Build history of the part. All positions in model axes, mm. Face numbers are marked on the shaded views. A direction names the side the tool comes from. Give positions to 0.01 mm unless a question says otherwise; leave off trailing zeros. Order: outer loops, then holes, each group sorted by start corner. A loop starts at its lowest first (then second) coordinate and runs counter-clockwise, first axis right, second up. Notation, with made-up numbers: (82.5, 29) - (121.5, 29) arc R25 ccw to (121.5, 68) - close; hole circle Ø8 at (-31, 84.25). An arc over 180 degrees is marked (long way). Write each question's results on one line, items separated by ' | '. Start each with the question number.
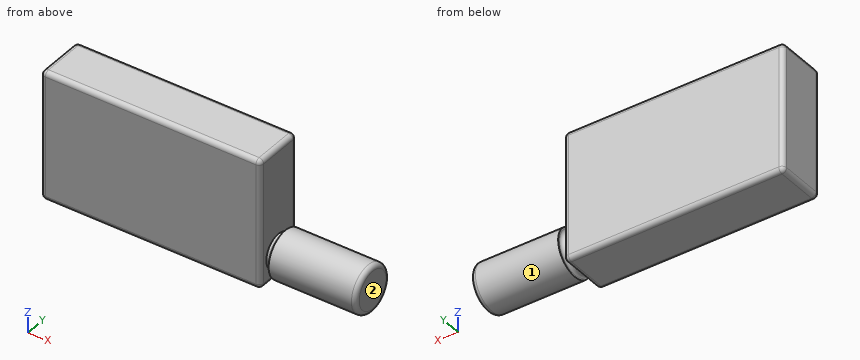
from build123d import *

# Parameters (mm, degrees)
SKETCH1_W           = 48
SKETCH1_H           = 28.2
BOSS_EXTRUDE1_DEPTH = 11
SKETCH2_R           = 3.7
BOSS_EXTRUDE2_DEPTH = 1.5
SKETCH3_R           = 5.1
BOSS_EXTRUDE3_DEPTH = 19.1
FILLET1_R           = 1
FILLET2_R           = 1
FILLET3_R           = 1


with BuildPart() as part:
    # Sketch1 → Boss-Extrude1 (new body)
    with BuildSketch(Plane(origin=(0, 0, 0), x_dir=(1, 0, 0), z_dir=(0, 1, 0))):
        with Locations((24, 14.1)):
            Rectangle(SKETCH1_W, SKETCH1_H)
    extrude(amount=BOSS_EXTRUDE1_DEPTH)

    # Sketch2 → Boss-Extrude2 (add)
    with BuildSketch(Plane(origin=(48, 0, 0), x_dir=(0, 0, -1), z_dir=(1, 0, 0))):
        with Locations((22.7, 5.5)):
            Circle(SKETCH2_R)
    extrude(amount=BOSS_EXTRUDE2_DEPTH)

    # Sketch3 → Boss-Extrude3 (add)
    with BuildSketch(Plane(origin=(49.5, 0, 0), x_dir=(0, 0, -1), z_dir=(1, 0, 0))):
        with Locations((22.7, 5.5)):
            Circle(SKETCH3_R)
    extrude(amount=BOSS_EXTRUDE3_DEPTH)

    # Fillet1
    fillet1_edges = [part.edges().sort_by_distance(p)[0] for p in [
        (48, 11, -14.1),
        (24, 11, -28.2),
        (0, 11, -14.1),
        (24, 0, -28.2),
        (48, 0, -14.1),
        (24, 0, 0),
        (0, 0, -14.1),
        (0, 5.5, -28.2),
        (48, 5.5, -28.2),
        (48, 5.5, 0),
        (0, 5.5, 0),
        (24, 11, 0),
    ]]
    fillet(fillet1_edges, radius=FILLET1_R)

    # Fillet2
    fillet2_edges = [part.edges().sort_by_distance(p)[0] for p in [
        (68.6, 5.5, -17.6),
    ]]
    fillet(fillet2_edges, radius=FILLET2_R)

    # Fillet3
    fillet3_edges = [part.edges().sort_by_distance(p)[0] for p in [
        (49.5, 5.5, -19),
    ]]
    fillet(fillet3_edges, radius=FILLET3_R)


solid = part.part
Item 1: Flat gauge pin, fed straight in: pin 1 Ø4.5 at (y, z) = (7.5, -8.5) entering from +X. Where does the tip first touch, or does it go through?
Item 2: Cut at C-C, the plane z = -22.7. List the corners of the cut face in (x, y), then the cut area to 3 significant figures.
Item 3: Cut at B-B, the plane y = 5.5. List the corners of the cut face in (x, z).
Item 4: Cut at A-A, the plane z = -2.5. List the corners of the cut face in (x, y), then the cut area to 3 significant figures.
Item 5: Cut at D-D, the plane x = 56. List the corners of the cut face in (y, z).
Item 6: Which spindle directions (+Z, -Z, +X, -X, +Y, -Y) get a long thin tool onto all of the face, cutting with end or side? Do the marked faces 1 and 2. Say none if no direction does.
Item 7: Probe line 1 along X through (y, z) = (6, -7.25); line 2 along Z through (x, y) = (57, 5.75); line 3 along Z through (x, y) = (47.5, 8.5). List the from-to ranges inside material, lowest first. Write a range as from..to.
Values found:
1) pin 1: stops at x = 48
2) outline: (0, 1) arc R1 ccw to (1, 0) - (47, 0) arc R1 ccw to (48, 1) - (48, 1.8) - (48.5, 1.8) arc R1 cw to (49.5, 0.8) - (49.5, 0.4) - (67.6, 0.4) arc R1 ccw to (68.6, 1.4) - (68.6, 9.6) arc R1 ccw to (67.6, 10.6) - (49.5, 10.6) - (49.5, 10.2) arc R1 cw to (48.5, 9.2) - (48, 9.2) - (48, 10) arc R1 ccw to (47, 11) - (1, 11) arc R1 ccw to (0, 10) - close | area: 733 mm2
3) outline: (0, -27.2) arc R1 ccw to (1, -28.2) - (47, -28.2) arc R1 ccw to (48, -27.2) - (48, -26.4) - (48.5, -26.4) arc R1 cw to (49.5, -27.4) - (49.5, -27.8) - (67.6, -27.8) arc R1 ccw to (68.6, -26.8) - (68.6, -18.6) arc R1 ccw to (67.6, -17.6) - (49.5, -17.6) - (49.5, -18) arc R1 cw to (48.5, -19) - (48, -19) - (48, -1) arc R1 ccw to (47, 0) - (1, 0) arc R1 ccw to (0, -1) - close
4) outline: (0, 1) arc R1 ccw to (1, 0) - (47, 0) arc R1 ccw to (48, 1) - (48, 10) arc R1 ccw to (47, 11) - (1, 11) arc R1 ccw to (0, 10) - close | area: 527 mm2
5) outline: circle Ø10.2 at (5.5, -22.7)
6) face 1: +X | face 2: +Z, -Z, +X, +Y, -Y
7) line 1: x = 0..48 | line 2: z = -27.79..-17.61 | line 3: z = -28.07..-0.13
